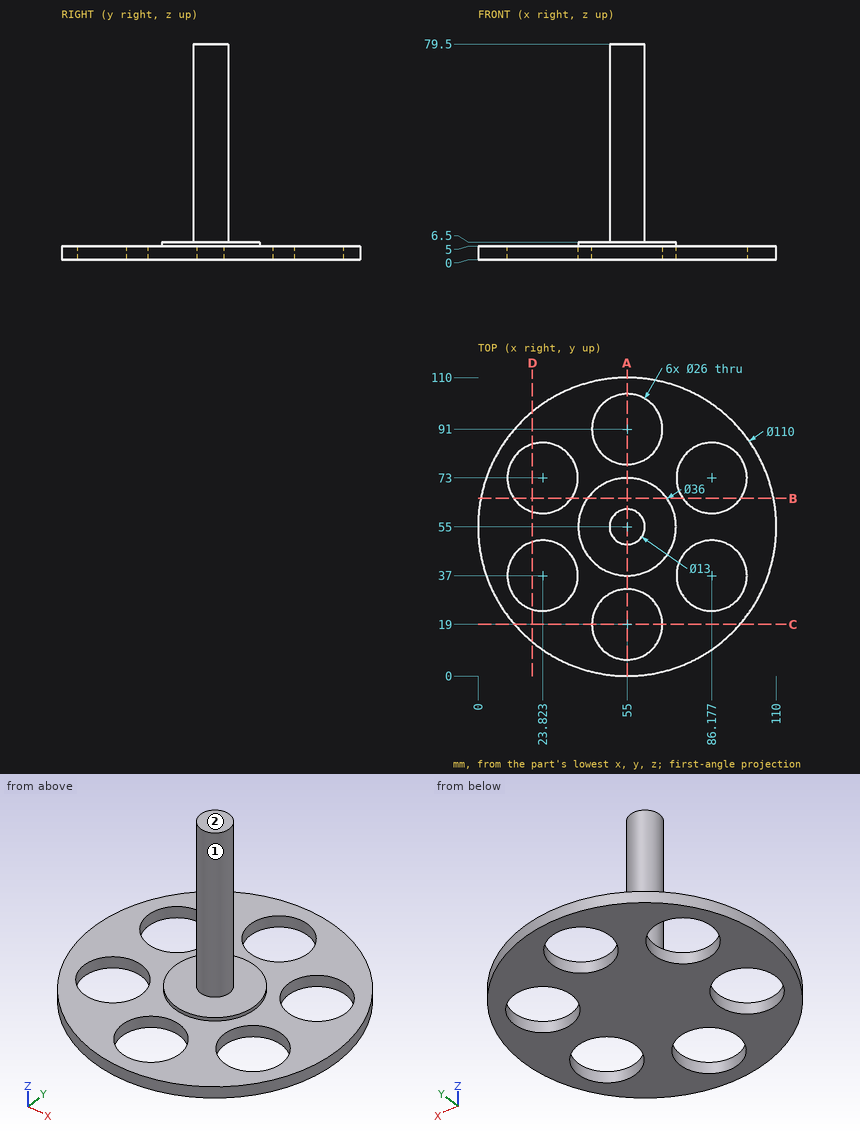
Can you work these out from the drawing? Everything is in mm from the part's minimum corner. A direction names the side the tool comes from. Give positions to 0.01 mm unless a question says otherwise; leave off trailing zeros. Loops run counter-clockwise (first coordinate to the right, second up) from the corner with the lowest first, then second, coordinate; pieces in that order, holes last. Notation, with made-up numbers: (83.5, -35.5) -> (109.5, -35.5) arc R35 ccw to (109.5, 1.5) -> close; hole circle Ø10 at (-25, -37). An arc over 180 degrees is marked (long way). Put each result on its own line as item: value.
(1) Imagine slicing it at D-D on x = 20. Write out the boundary of the cut face in (y, z) (1 decimal).
Computed:
outline: (12.6, 0) -> (24.6, 0) -> (24.6, 5) -> (12.6, 5) -> close; (49.4, 0) -> (60.6, 0) -> (60.6, 5) -> (49.4, 5) -> close; (85.4, 0) -> (97.4, 0) -> (97.4, 5) -> (85.4, 5) -> close
(2) Imagine slicing it at A-A on x = 55. Write out the boundary of the cut face in (y, z), plus the area to 3 significant figures.
Computed:
outline: (0, 0) -> (6, 0) -> (6, 5) -> (0, 5) -> close; (32, 0) -> (78, 0) -> (78, 5) -> (73, 5) -> (73, 6.5) -> (61.5, 6.5) -> (61.5, 79.5) -> (48.5, 79.5) -> (48.5, 6.5) -> (37, 6.5) -> (37, 5) -> (32, 5) -> close; (104, 0) -> (110, 0) -> (110, 5) -> (104, 5) -> close
area: 1,290 mm^2
(3) Imagine slicing it at C-C on y = 19. Write out the boundary of the cut face in (x, z).
Computed:
outline: (13.42, 0) -> (42, 0) -> (42, 5) -> (13.42, 5) -> close; (68, 0) -> (96.58, 0) -> (96.58, 5) -> (68, 5) -> close
(4) I'm going to push flat-ended pins straight in: pin 1 Ø21 at (x, y) = (55, 19) entering from -Z; pin 2 Ø1.5 at (y, z) = (59.5, 30) entering from -X; pin 3 Ø6 at (x, z) = (50.5, 58) entering from -Y; pin 4 Ø12 at (x, z) = (44, 46) entering from +Y. Where does each tip first touch, or does it pass through?
Computed:
pin 1: through
pin 2: x = 49.69
pin 3: y = 48.68
pin 4: y = 59.15
(5) For the marked faces 1 and 2, which set-ups out of +Z, -Z, +X, -X, +Y, -Y let a thin tool reach every point of the face, with its end or its side?
Computed:
face 1: +Z
face 2: +Z, +X, -X, +Y, -Y
(6) Imagine slicing it at B-B on y = 65.5. Write out the boundary of the cut face in (x, z), plus the area to 3 significant figures.
Computed:
outline: (1.01, 0) -> (13.2, 0) -> (13.2, 5) -> (1.01, 5) -> close; (34.44, 0) -> (75.56, 0) -> (75.56, 5) -> (69.62, 5) -> (69.62, 6.5) -> (40.38, 6.5) -> (40.38, 5) -> (34.44, 5) -> close; (96.8, 0) -> (108.99, 0) -> (108.99, 5) -> (96.8, 5) -> close
area: 371 mm^2
(7) Please list where these lines run through material, in increasing order: probe 1 along Y at (x, z) = (55, 2.9); probe 2 along Z at (x, y) = (7, 63.5); probe 3 along Z at (x, y) = (71, 63). Write a range as [from, to].
Computed:
probe 1: [0, 6], [32, 78], [104, 110]
probe 2: [0, 5]
probe 3: [0, 6.5]
